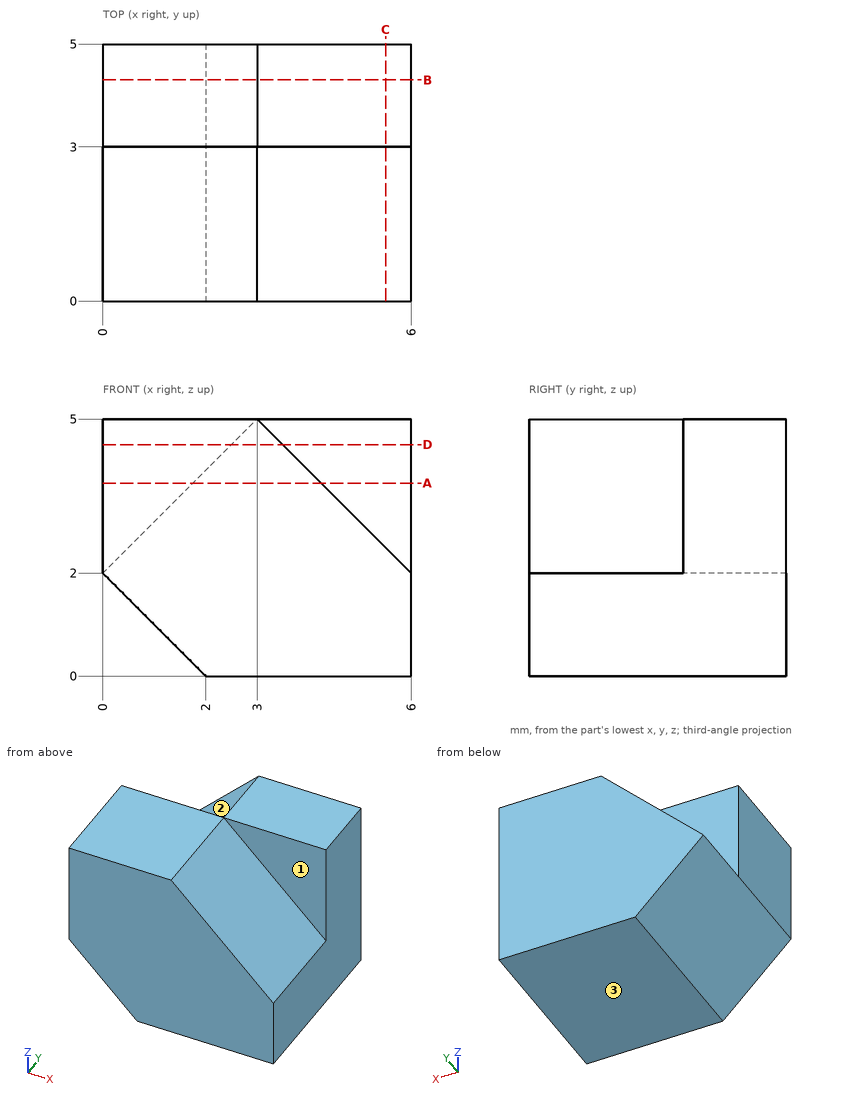
Check sheet for the drawn part. Datum: minimum x, y, z corner. Units: mm. A direction names the side the tool comes from. Coordinates: 2 decimals unless noted, no trailing zeros. Order: outer loops, then holes, each group sorted by start corner. A loop starts at its lowest first (then second) coordinate and runs counter-clockwise, first axis right, second up. Notation, with made-up numbers: (-40, 11.5) - (14, 11.5) arc R18 cw to (14, 27.5) - close; hole circle Ø11 at (54, 66). An arc over 180 degrees is marked (long way). Return JSON: item names as keys, results as strings.
(1) Section check B-B, the plane y = 4.3. Record the cut outline in (x, z).
Filled sheet:
{"outline": "(0, 2) - (2, 0) - (6, 0) - (6, 5) - (3, 5) - close"}
(2) Section check D-D, the plane z = 4.5. Record the cut outline in (x, y), and give its area (3 significant figures).
Filled sheet:
{"outline": "(0, 0) - (3.5, 0) - (3.5, 3) - (6, 3) - (6, 5) - (2.5, 5) - (2.5, 3) - (0, 3) - close", "area": "17.5 mm^2"}
(3) Section check C-C, the plane x = 5.5. Record the cut outline in (y, z).
Filled sheet:
{"outline": "(0, 0) - (5, 0) - (5, 5) - (3, 5) - (3, 2.5) - (0, 2.5) - close"}
(4) Thickness scan on line 1 along Y through (x, z) = (1.05, 3.7); line 2 along Z through (x, y) = (2.95, 3.25); line 3 along X through (y, z) = (0.5, 1.8). Record the ranges inside material, lowest first.
Filled sheet:
{"line 1": "y = 0 to 3", "line 2": "z = 0 to 4.95", "line 3": "x = 0.2 to 6"}
(5) Section check A-A, the plane z = 3.75. Record the cut outline in (x, y).
Filled sheet:
{"outline": "(0, 0) - (4.25, 0) - (4.25, 3) - (6, 3) - (6, 5) - (1.75, 5) - (1.75, 3) - (0, 3) - close"}
(6) Access from +Z, -Z, +X, -X, +Y, -Y to the whole of each face (thin tool, end or side, straight path). Record for the marked faces 1, 2 and 3.
Filled sheet:
{"face 1": "+Z, +X, -Y", "face 2": "+Z, -X, +Y", "face 3": "-Z, +X, -X, +Y, -Y"}
